Part model, mm, in its own coordinate system. A direction names the side the tool comes from. Coordinates: 2 decimals unless noted, no trailing zeros. Loops run counter-clockwise (first coordinate to the right, second up) from the corner with the lowest first, then second, coordinate; pieces in that order, holes last. Notation, with made-up numbers: M 47,30.25 L 96,30.25 A16 cw 96,50.25 Z; hole C -36.75,60 d6. An arc over 180 degrees is marked long. Answer as a JSON object with one key per item and string values. Group by question number.
1. 3-axis set-ups, long thin cutter, end or side, ignore diameter. For faces 1 (the face through (0, -14, 0)), 2 (the face through (2, -1, 2)): which of +Z, -Z, +X, -X, +Y, -Y reach the whole face in a straight line?
2. Saw through at B-B on x = 0. Write the cut outline in (y, z), then the cut area to 3 significant figures.
3. Saw through at D-D on y = 16.5. Write the cut outline in (x, z), then the cut area to 3 significant figures.
4. Saw through at A-A on z = 0. Write the cut outline in (x, y), then the cut area to 3 significant figures.
5. Drill centre lines: L1, parallel to Z at x = 2, y = -5.5; L2, parallel to X at y = 7.5, z = -2.5; L3, parallel to Y at x = 1, z = -10.25. Where is each one in solid material? Low to high.
6. Drop flat-ended pins along their axis: pin 1 Ø3 at (x, y) = (-1.5, 6.5) entering from +Z; pin 2 Ø12 at (x, y) = (-4.5, -10) entering from -Z; pin 3 Ø8 at (x, z) = (6, 5) entering from -Y; pin 4 Ø10 at (x, y) = (11, -4) entering from -Z. Give the stop position or say it passes through.
7. Saw through at C-C on y = -8. Write the cut outline in (x, z), then the cut area to 3 significant figures.
from build123d import *

# Parameters (mm, degrees)
SKETCH1_R           = 14
BOSS_EXTRUDE4_DEPTH = 19
SKETCH7_R           = 2.25
BOSS_EXTRUDE5_DEPTH = 14
SKETCH9_R           = 4
BOSS_EXTRUDE8_DEPTH = 1


with BuildPart() as part:
    # Sketch1 → Boss-Extrude4 (new body)
    with BuildSketch(Plane(origin=(0, 0, 0), x_dir=(1, 0, 0), z_dir=(0, 1, 0))):
        with Locations(Location((0, 0, 0), (0, 0, 270))):
            Circle(SKETCH1_R)
    extrude(amount=BOSS_EXTRUDE4_DEPTH)

    # Sketch7 → Boss-Extrude5 (add)
    with BuildSketch(Plane.XZ):
        with Locations(Location((0, 0, 0), (0, 0, 270))):
            Circle(SKETCH7_R)
    extrude(amount=BOSS_EXTRUDE5_DEPTH)

    # Sketch9 → Boss-Extrude8 (add)
    with BuildSketch(Plane.XZ):
        with Locations(Location((0, 0, 0), (0, 0, 90))):
            Circle(SKETCH9_R)
    extrude(amount=BOSS_EXTRUDE8_DEPTH)

    # Sketch10 → Cut-Revolve9 (revolve, cut)
    with BuildSketch(Plane.XY, mode=Mode.PRIVATE) as cut_revolve9_sk:
        Polygon((-4, 0), (-14, 0), (-14, 1.001232808), (-13.499383596, 0.500616404), align=None)
    revolve(cut_revolve9_sk.sketch.rotate(Axis((0, 0.500616404, 0), (0, 1, 0)), 90), axis=Axis((0, 0.500616404, 0), (0, 1, 0)), mode=Mode.SUBTRACT)


solid = part.part
Outcome:
{
 "1": {"face 1": "+Z, -Z, +X, -X, -Y", "face 2": "-Y"},
 "2": {"outline": "M -14,-2.25 L -1,-2.25 L -1,-4 L 0,-4 L 0.5,-13.5 L 1,-14 L 19,-14 L 19,14 L 1,14 L 0.5,13.5 L 0,4 L -1,4 L -1,2.25 L -14,2.25 Z", "area": "593 mm²"},
 "3": {"outline": "C 0,0 d28", "area": "616 mm²"},
 "4": {"outline": "M -14,1 L -13.5,0.5 L -4,0 L -4,-1 L -2.25,-1 L -2.25,-14 L 2.25,-14 L 2.25,-1 L 4,-1 L 4,0 L 13.5,0.5 L 14,1 L 14,19 L -14,19 Z", "area": "593 mm²"},
 "5": {"L1": "z = -1.03 to 1.03", "L2": "x = -13.77 to 13.77", "L3": "y = 0.33 to 19"},
 "6": {"pin 1": "stops at z = 14", "pin 2": "stops at z = -2.25", "pin 3": "stops at y = -1", "pin 4": "stops at z = -10.22"},
 "7": {"outline": "C 0,0 d4.5", "area": "15.9 mm²"}
}
